Could you check a few things on this model? Use its own coordinates, in mm. Face numbers are marked on the shaded views. Give positions to 0.01 mm unless a question says otherwise; leave off trailing zeros. Write each loop counter-clockwise with the first axis right and the second up, starting at its lowest first coordinate (ties: lowest second). Pieces come first, ordered by that corner, then holes. Notation, with made-up numbers: (52.5, 29.25) - (60.5, 29.25) arc R23 cw to (60.5, 63.25) - close; hole circle Ø7 at (-30, 74.25). An arc over 180 degrees is marked (long way). Answer in a Markdown table with one row per item.
Autodesk Inventor part; units mm, degrees
ref_plane "YZ Plane" through (0, 0, 0) normal (1, 0, 0) x (0, 1, 0)
ref_plane "XZ Plane" through (0, 0, 0) normal (0, 1, 0) x (-1, 0, 0)
ref_plane "XY Plane" through (0, 0, 0) normal (0, 0, 1) x (1, 0, 0)
sketch "스케치1" plane through (0, 0, 0) normal (0, 1, 0) x (-1, 0, 0)
  line L0 (0, 0) -> (-90, 0)
  line L1 (-90, 0) -> (-90, -130)
  line L2 (-90, -130) -> (0, -130)
  line L3 (0, -130) -> (0, 0)
  dimension "d0" = 90
  dimension "d1" = 130
extrude "돌출1" add sketch "스케치1" along normal blind 2
sketch "스케치2" plane through (0, 2, 0) normal (0, 1, 0) x (1, 0, 0)
  circle A0 centre (85, 95) radius 5
  circle A1 centre (85, 35) radius 5
  line L0 (0, 0) -> (90, 0)
  line L1 (90, 0) -> (90, 130)
  line L2 (90, 130) -> (0, 130)
  line L3 (0, 130) -> (0, 0)
  circle A2 centre (15, 105) radius 5
  circle A3 centre (15, 95) radius 5
  circle A4 centre (15, 35) radius 5
  circle A5 centre (15, 25) radius 5
  dimension "d4" = 10
  dimension "d5" = 10
  dimension "d6" = 5
  dimension "d7" = 5
  dimension "d8" = 35
  dimension "d9" = 35
  dimension "d10" = 10
  dimension "d11" = 10
  dimension "d12" = 10
  dimension "d13" = 10
  dimension "d14" = 25
  dimension "d15" = 10
  dimension "d16" = 25
  dimension "d17" = 10
  dimension "d18" = 15
  dimension "d19" = 15
  dimension "d20" = 15
  dimension "d21" = 15
extrude "돌출2" add sketch "스케치2" along normal blind 13 contours A0 | A1 | A2 | A3 | A4 | A5
sketch "스케치3" plane through (0, 2, 0) normal (0, 1, 0) x (1, 0, 0)
  circle A0 centre (87, 127) radius 1.5
  circle A1 centre (87, 65) radius 1.5
  circle A2 centre (87, 3) radius 1.5
  line L0 (90, 0) -> (90, 130)
  line L1 (90, 130) -> (0, 130)
  line L2 (0, 0) -> (90, 0)
  circle A3 centre (3, 127) radius 1.5
  circle A4 centre (3, 3) radius 1.5
  line L3 (0, 130) -> (0, 0)
  dimension "d24" = 3
  dimension "d25" = 3
  dimension "d26" = 3
  dimension "d27" = 3
  dimension "d28" = 3
  dimension "d29" = 3
  dimension "d30" = 3
  dimension "d31" = 3
  dimension "d32" = 62
  dimension "d33" = 3
  dimension "d34" = 3
  dimension "d35" = 3
  dimension "d36" = 3
  dimension "d37" = 3
  dimension "d38" = 3
extrude "돌출3" cut sketch "스케치3" against normal blind 2 contours A0 | A1 | A2 | A3 | A4
properties part number "13090모터드라이브"
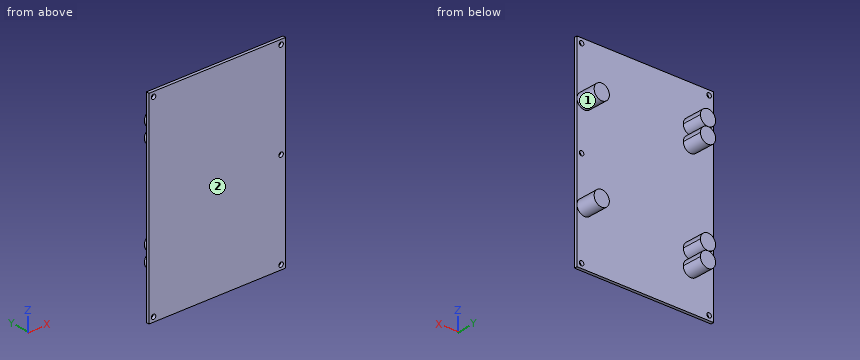
1) Imagine slicing it at C-C (z = -3). List the corners of the cut face in (x, y) for me.
Check values:
| item | result |
|---|---|
| outline | (0, 0) - (1.5, 0) - (1.5, 2) - (0, 2) - close; (4.5, 0) - (85.5, 0) - (85.5, 2) - (4.5, 2) - close; (88.5, 0) - (90, 0) - (90, 2) - (88.5, 2) - close |
2) Will these pins go through, and if not, where does the flat tip stop? P1, Ø1, axis at x = 69.5, z = -33, coming from the +Y side; P2, Ø2, axis at y = 11.5, z = -31, coming from the +X side.
Check values:
| item | result |
|---|---|
| P1 | stops at y = 2 |
| P2 | stops at x = 89 |
3) If I drill on line 1 (Z direction, x = 87, y = 1.65); line 2 (X direction, y = 0.85, z = -127); line 3 (X direction, y = 0.75, z = -65), over which ranges is the centre line in solid material (lowest first)?
Check values:
| item | result |
|---|---|
| line 1 | z = -130 to -128.5, -125.5 to -66.5, -63.5 to -4.5, -1.5 to 0 |
| line 2 | x = 0 to 1.5, 4.5 to 85.5, 88.5 to 90 |
| line 3 | x = 0 to 85.5, 88.5 to 90 |
4) We'd pull the mould along X, two halves only. Please class the marked faces 1 and 2: +X half, -X half, draft (parallel to the pull), parting line (faces both ways), or undercut.
Check values:
| item | result |
|---|---|
| face 1 | undercut |
| face 2 | draft |
5) Imagine slicing it at A-A (x = 3). List the corners of the cut face in (y, z) for me.
Check values:
| item | result |
|---|---|
| outline | (0, -130) - (2, -130) - (2, -128.5) - (0, -128.5) - close; (0, -125.5) - (2, -125.5) - (2, -4.5) - (0, -4.5) - close; (0, -1.5) - (2, -1.5) - (2, 0) - (0, 0) - close |
6) Imagine slicing it at D-D (x = 87). List the corners of the cut face in (y, z) for me, then the cut area to 3 significant figures.
Check values:
| item | result |
|---|---|
| outline | (0, -130) - (2, -130) - (2, -128.5) - (0, -128.5) - close; (0, -125.5) - (2, -125.5) - (2, -99.58) - (15, -99.58) - (15, -90.42) - (2, -90.42) - (2, -66.5) - (0, -66.5) - close; (0, -63.5) - (2, -63.5) - (2, -39.58) - (15, -39.58) - (15, -30.42) - (2, -30.42) - (2, -4.5) - (0, -4.5) - close; (0, -1.5) - (2, -1.5) - (2, 0) - (0, 0) - close |
| area | 480 mm2 |
